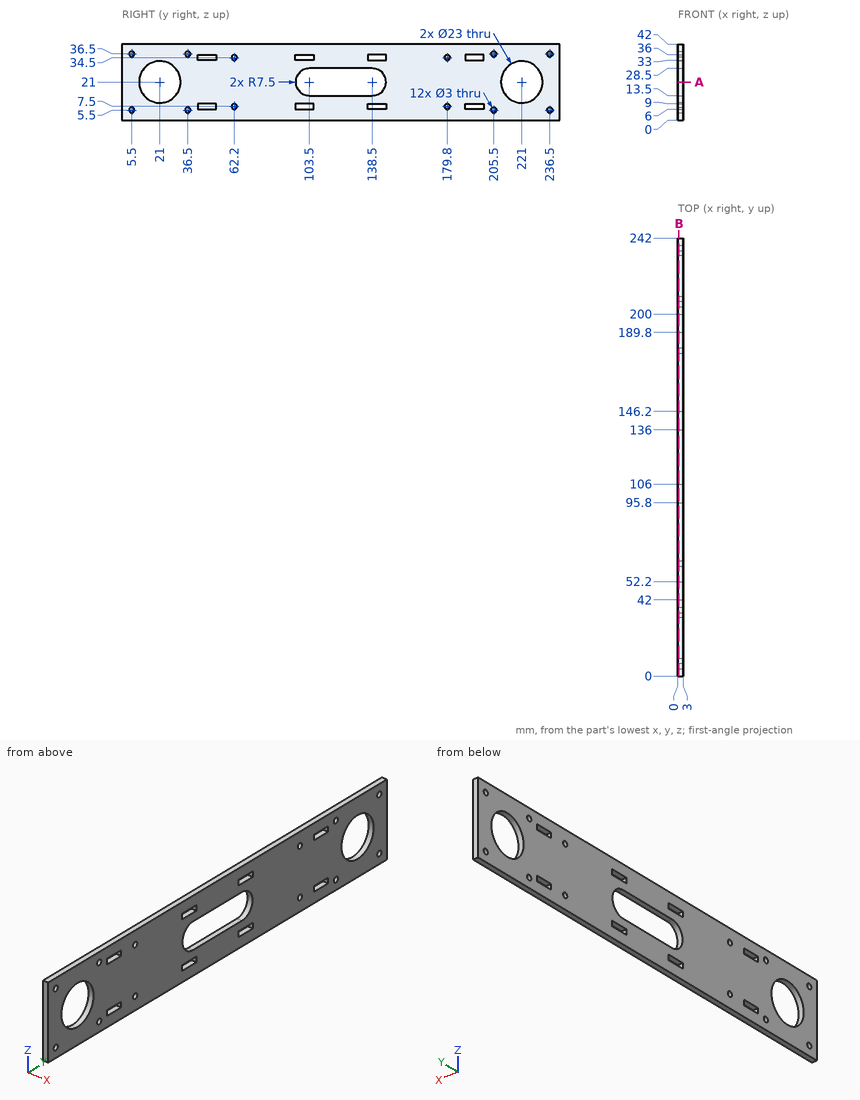
Study the drawing (mm; zero at the part's minimum x, y, z) and answer. Give positions to 0.01 mm unless a question says otherwise; leave off trailing zeros. Order: outer loops, then holes, each group sorted by start corner. A loop starts at its lowest first (then second) coordinate and runs counter-clockwise, first axis right, second up. Notation, with made-up numbers: (57, -16.75) -> (105, -16.75) arc R20 ccw to (105, 14.25) -> close; hole circle Ø9 at (68, -8). An arc over 180 degrees is marked (long way). Put each result on its own line as item: value.
Item 1: A cutting plane is placed at A-A on z = 21. Give the vertices of the cut face in (x, y).
Established:
outline: (0, 0) -> (3, 0) -> (3, 9.5) -> (0, 9.5) -> close; (0, 32.5) -> (3, 32.5) -> (3, 96) -> (0, 96) -> close; (0, 146) -> (3, 146) -> (3, 209.5) -> (0, 209.5) -> close; (0, 232.5) -> (3, 232.5) -> (3, 242) -> (0, 242) -> close
Item 2: Straight lines are drawn through the part: line 1 (Z direction, x = 1.05, y = 190.5); line 2 (Z direction, x = 0.35, y = 138); line 3 (Y direction, x = 1.5, z = 20.5). For each, find the intervals that lie inside material, in ascending order.
Established:
line 1: z = 0 to 6, 9 to 33, 36 to 42
line 2: z = 0 to 6, 9 to 13.5, 28.5 to 33, 36 to 42
line 3: y = 0 to 9.51, 32.49 to 96.02, 145.98 to 209.51, 232.49 to 242
Item 3: A cutting plane is placed at B-B on x = 0.6. Count the separate pieces of the cut face and the enclosed holes in it, plus the area to 3 significant figures.
Established:
separate pieces: 1
enclosed holes: 23
area: 8,300 mm^2
